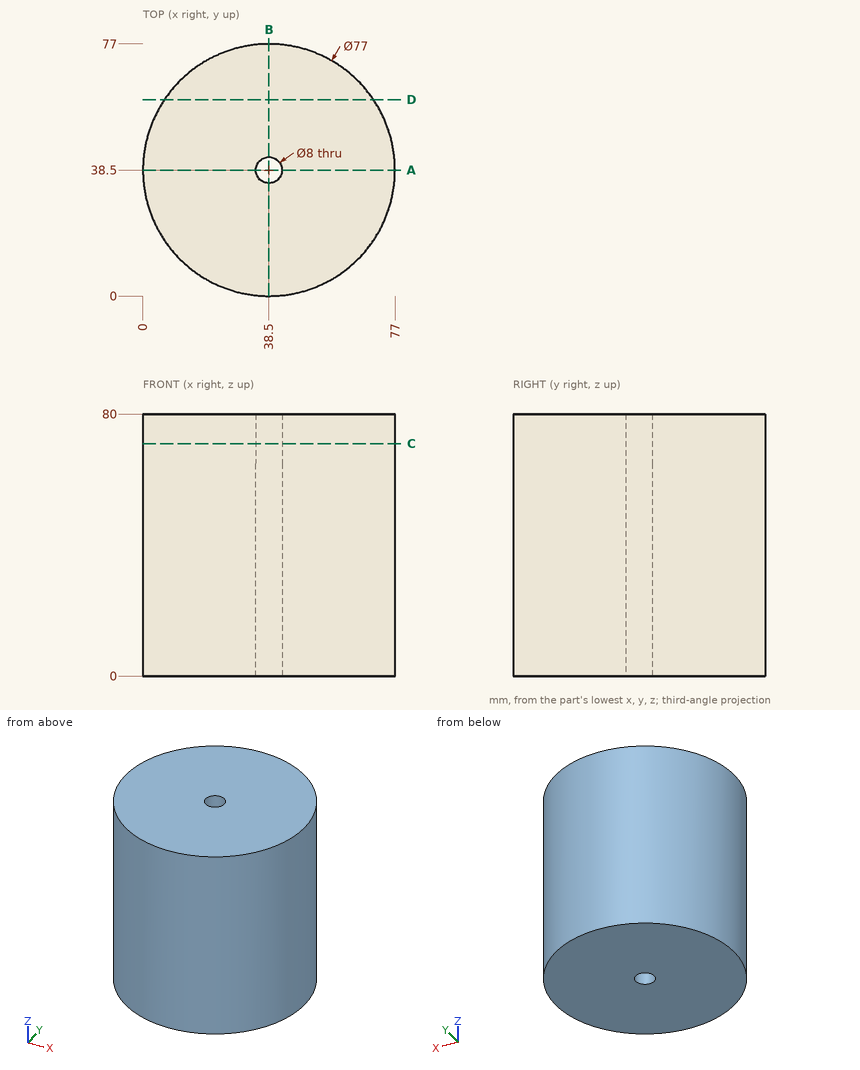
Geometry: see drawing. Coordinates: mm, zero at the bounding-box minimum. Round coordinates to 2 decimals unless told otherwise and drop trailing zeros. Loops run counter-clockwise (first coordinate to the right, second up) from the corner with the lowest first, then second, coordinate; pieces in that order, holes last. Notation, with made-up numbers: (77, 52.5) -> (131, 52.5) arc R20 cw to (131, 64.5) -> close; hole circle Ø1 at (46.25, 6). An arc over 180 degrees is marked (long way). One line per question, with ' | ' between items. Start each with the question number.
1. Section C-C on z = 71. Output: boundary loops of the cut face in (x, y), and give its area (3 significant figures).
2. Line query: line 1 along Y through (x, z) = (38.5, 56.5); line 2 along X through (y, z) = (42, 30); line 3 along X through (y, z) = (38, 47). Output: solid intervals per line, ascending. Write a range as [from, to].
3. Section A-A on y = 38.5. Output: boundary loops of the cut face in (x, z), and give its area (3 significant figures).
4. Section D-D on y = 60. Output: boundary loops of the cut face in (x, z), and give its area (3 significant figures).
5. Contact query for flat-ended pins moving along their axis: pin 1 (1 mm diameter, centred on x = 50, z = 60.5, fed in from +Y); pin 2 (8 mm diameter, centred on x = 45.5, z = 19.5, fed in from +Y); pin 3 (10 mm diameter, centred on y = 57, z = 66, fed in from +X). Output: stop coordinate, or through.
Returned:
1) outline: circle Ø77 at (38.5, 38.5); hole circle Ø8 at (38.5, 38.5) | area: 4,610 mm2
2) line 1: y = [0, 34.5], [42.5, 77] | line 2: x = [0.16, 36.56], [40.44, 76.84] | line 3: x = [0, 34.53], [42.47, 77]
3) outline: (0, 0) -> (34.5, 0) -> (34.5, 80) -> (0, 80) -> close; (42.5, 0) -> (77, 0) -> (77, 80) -> (42.5, 80) -> close | area: 5,520 mm2
4) outline: (6.56, 0) -> (70.44, 0) -> (70.44, 80) -> (6.56, 80) -> close | area: 5,110 mm2
5) pin 1: stops at y = 75.4 | pin 2: stops at y = 76.88 | pin 3: stops at x = 74.56
